```python
from build123d import *

# Parameters (mm, degrees)
PAD001_DEPTH                               = 15
SKETCH007_R                                = 1.65
POCKET005_DEPTH                            = 7.001
SKETCH008_R                                = 3.2
POCKET006_DEPTH                            = 3
CHAMFER004013007011015006009007001025_SIZE = 4
CHAMFER004013007011015006009007001026_SIZE = 0.4
CHAMFER004013007011015006009007001027_SIZE = 1
SKETCH009_W                                = 3
SKETCH009_H                                = 3.2
PAD002_DEPTH                               = 1


with BuildPart() as part:
    # Sketch006 → Pad001 (new body)
    with BuildSketch(Plane.XY):
        Polygon((-5, 0), (-5, 3), (-3, 5), (3, 5), (5, 3), (5, 0), (15, 0), (15, 5), (15, 7), (-15, 7), (-15, 6), (-15, 0), align=None)
    extrude(amount=PAD001_DEPTH)

    # Sketch007 (on Face12 of Pad001) → Pocket005 (cut, through all)
    with BuildSketch(Plane.XZ):
        with Locations((-10, 7.5)):
            Circle(SKETCH007_R)
        with Locations((10, 7.5)):
            Circle(SKETCH007_R)
    extrude(amount=-POCKET005_DEPTH, mode=Mode.SUBTRACT)

    # Sketch008 (on Face14 of Pocket005) → Pocket006 (cut)
    with BuildSketch(Plane(origin=(0, 7, 0), x_dir=(-1, 0, 0), z_dir=(0, 1, 0))):
        with Locations((-10, 7.5)):
            Circle(SKETCH008_R)
        with Locations((10, 7.5)):
            Circle(SKETCH008_R)
    extrude(amount=-POCKET006_DEPTH, mode=Mode.SUBTRACT)

    # Chamfer004013007011015006009007001025
    chamfer004013007011015006009007001025_edges = [part.edges().sort_by_distance(p)[0] for p in [
        (15, 2.5, 15),
        (15, 2.5, 0),
        (15, 6, 0),
        (15, 6, 15),
        (-15, 3, 15),
        (-15, 6.5, 15),
        (-15, 6.5, 0),
        (-15, 3, 0),
    ]]
    chamfer(chamfer004013007011015006009007001025_edges, length=CHAMFER004013007011015006009007001025_SIZE)

    # Chamfer004013007011015006009007001026
    chamfer004013007011015006009007001026_edges = [part.edges().sort_by_distance(p)[0] for p in [
        (-15, 7, 7.5),
        (-13, 7, 2),
        (-13, 7, 13),
        (0, 7, 0),
        (0, 7, 15),
        (13, 7, 2),
        (13, 7, 13),
        (15, 7, 7.5),
        (-6.8, 7, 7.5),
        (13.2, 7, 7.5),
    ]]
    chamfer(chamfer004013007011015006009007001026_edges, length=CHAMFER004013007011015006009007001026_SIZE)

    # Chamfer004013007011015006009007001027
    chamfer004013007011015006009007001027_edges = [part.edges().sort_by_distance(p)[0] for p in [
        (-5, 1.5, 15),
        (-4, 4, 15),
        (0, 5, 15),
        (4, 4, 15),
        (5, 1.5, 15),
        (-5, 1.5, 0),
        (-4, 4, 0),
        (0, 5, 0),
        (4, 4, 0),
        (5, 1.5, 0),
    ]]
    chamfer(chamfer004013007011015006009007001027_edges, length=CHAMFER004013007011015006009007001027_SIZE)

    # Sketch009 (on Face13 of Chamfer004013007011015006009007001027) → Pad002 (join)
    with BuildSketch(Plane.XZ):
        with Locations((-13.5, 7.5)):
            Rectangle(SKETCH009_W, SKETCH009_H)
        with Locations((-6.5, 7.5)):
            Rectangle(SKETCH009_W, SKETCH009_H)
        with Locations((6.5, 7.5)):
            Rectangle(SKETCH009_W, SKETCH009_H)
        with Locations((13.5, 7.5)):
            Rectangle(SKETCH009_W, SKETCH009_H)
    extrude(amount=PAD002_DEPTH)


solid = part.part
```
Work out the finished part from the listing and answer in its coordinate system (mm). A direction names the side the tool comes from. Round coordinates to 2 decimals unless told otherwise and drop trailing zeros. Write each loop counter-clockwise with the first axis right and the second up, starting at its lowest first coordinate (ties: lowest second). Pieces come first, ordered by that corner, then holes. Notation, with made-up numbers: (88, 28) -> (97, 28) arc R21 ccw to (97, 57) -> close; hole circle Ø9 at (53.5, -9). An arc over 180 degrees is marked (long way). Write each question's results on one line, items separated by ' | '.
1) Which of the six approach directions +Z, -Z, +X, -X, +Y, -Y give full straight-line access (tool end or side, diameter ignored) to faces 5 (the cylindrical face through (-9.306, 5.318, 4.376)), 6 (the flat face through (-13.5, -0.5, 5.9)), 7 (the flat face through (0, 5.5, 14.5)), 8 (the flat face through (6.5, -0.5, 9.1))?
Findings:
face 5: +Y | face 6: -Z, +X, -X, -Y | face 7: +Z, -Y | face 8: +Z, +X, -X, -Y
2) Flat-ended cylindrical pins translate along their axes: pin 1 (4.5 mm diameter, centred on x = -10, z = 7.5, fed in from +Y); pin 2 (3 mm diameter, centred on x = 1, z = 5, fed in from -Y); pin 3 (4 mm diameter, centred on x = -3, y = 2.5, fed in from -Z). Find the tip coordinate at first contact, or state that the pin passes through.
Findings:
pin 1: stops at y = 4 | pin 2: stops at y = 5 | pin 3: stops at z = 0.77
3) For a pull along X with two mould halves and no side action, classify faces 1 (the flat face through (-15, 3, 7)), 2 (the flat face through (-5.5, 1.7, 0.5)), 3 (the flat face through (-6.5, -0.5, 9.1)), 4 (the flat face through (5.5, 1.7, 14.5)) as +X half, -X half, draft (parallel to the pull), parting line (faces both ways), or undercut.
Findings:
face 1: -X half | face 2: undercut | face 3: draft | face 4: undercut
4) The part is cut by section A-A (y = 2.5). Write down the section's boundary in (x, z).
Findings:
outline: (-15, 4) -> (-11, 0) -> (-6, 0) -> (-5, 1) -> (-5, 14) -> (-6, 15) -> (-11, 15) -> (-15, 11) -> close; (5, 1) -> (6, 0) -> (11, 0) -> (15, 4) -> (15, 11) -> (11, 15) -> (6, 15) -> (5, 14) -> close; hole circle Ø3.3 at (-10, 7.5); hole circle Ø3.3 at (10, 7.5)
5) The part is cut by section C-C (z = 7.5). State how many separate pieces and enclosed holes the cut face has, and give its area (3 significant figures).
Findings:
separate pieces: 3 | enclosed holes: 0 | area: 111 mm²
6) The part is cut by section B-B (x = 10). Write down the section's boundary in (y, z), and give its area (3 significant figures).
Findings:
outline: (0, 0) -> (6.6, 0) -> (7, 0.4) -> (7, 3.9) -> (6.6, 4.3) -> (4, 4.3) -> (4, 5.85) -> (0, 5.85) -> close; (0, 9.15) -> (4, 9.15) -> (4, 10.7) -> (6.6, 10.7) -> (7, 11.1) -> (7, 14.6) -> (6.6, 15) -> (0, 15) -> close | area: 72.3 mm²
7) Consider line 1 along X through (y, z) = (4.75, 9.75); line 2 along X through (y, z) = (1, 9.5); line 3 along Z through (x, y) = (-10, 5.05). Determine where each line is inside the solid, lowest interval first. Write a range as [from, to].
Findings:
line 1: x = [-15, -12.28], [-7.72, -3.25], [3.25, 7.72], [12.28, 15] | line 2: x = [-15, -5], [5, 15] | line 3: z = [0, 4.3], [10.7, 15]
8) The part is cut by section D-D (x = 0.25). Write down the section's boundary in (y, z), and give its area (3 significant figures).
Findings:
outline: (5, 1) -> (6, 0) -> (6.6, 0) -> (7, 0.4) -> (7, 14.6) -> (6.6, 15) -> (6, 15) -> (5, 14) -> close | area: 28.8 mm²
